Verification items for the finished model (mm, model axes). Face numbers are marked on the shaded views. A direction names the side the tool comes from. Round coordinates to 2 decimals unless told otherwise and drop trailing zeros. Write each loop counter-clockwise with the first axis right and the second up, starting at its lowest first coordinate (ties: lowest second). Pieces come first, ordered by that corner, then holes. Notation, with made-up numbers: M 18,-9 L 63,-9 A28 cw 63,18 Z; hole C 7,2 d3. An arc over 180 degrees is marked long. One line per question, with ' | ' between items. Start each with the question number.
Q1. Gauge pin test, flat ends, axial feed: pin 1 (4 mm diameter, centred on x = 1.5, y = -3, fed in from +Z); pin 2 (10 mm diameter, centred on x = 27, y = 22.5, fed in from -Z); pin 3 (6 mm diameter, centred on y = 29, z = -5.5, fed in from +X). Record the tip position at first contact, or that the pin passes through.
Q2. Cross-section at B-B (z = 14.5). Record the boundary of the cut face in (x, y).
Q3. Release check for a two-part mould opening along X. For the marked faces 1 and 2 record: released by +X, released by -X, zero draft, split by the parting line, or undercut.
Q4. Cross-section at D-D (z = 0). Record the boundary of the cut face in (x, y).
Q5. Cross-section at A-A (y = 0). Record the boundary of the cut face in (x, z).
Q6. Cross-section at C-C (x = -26). Record the boundary of the cut face in (y, z), then the cut area to 3 significant figures.
Q7. Thickness scan on line 1 along Z through (x, y) = (-26, 32.75); line 2 along X through (y, z) = (34, 0); line 3 along Z through (x, y) = (-13, 0). Record the ranges inside material, lowest first. Write a range as from..to.
Q8. Tool access check on the marked faces 3 and 4. Record the directions out of +Z, -Z, +X, -X, +Y, -Y that give a thin tool (end or side, any length) a straight path to the whole face; none if there is none.
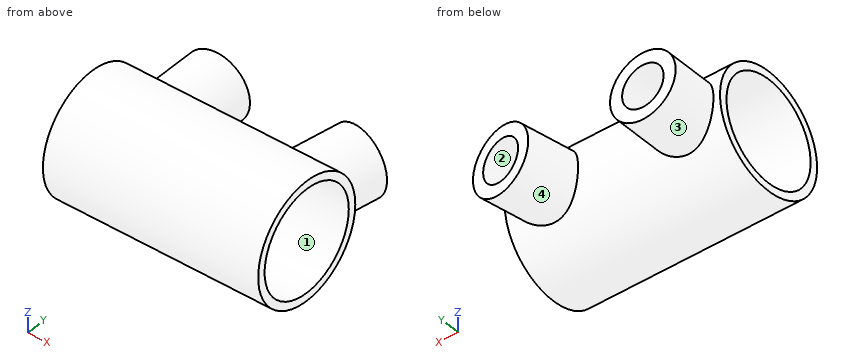
Autodesk Inventor part; units mm, degrees
ref_plane "Work Plane1" through (0, 40, 0) normal (0, 1, 0) x (-1, 0, 0)
ref_plane "Work Plane3" through (25, 40, 22.5) normal (0.1736, 0.9848, 0) x (0, 0, -1)
ref_plane "YZ Plane" through (0, 0, 0) normal (1, 0, 0) x (0, 1, 0)
sketch "Sketch1" plane through (0, 0, 0) normal (1, 0, 0) x (0, 1, 0)
  circle A0 centre (0, 0) radius 19.5
  circle A1 centre (0, 0) radius 22.5
  dimension "d0" = 39
  dimension "d1" = 45
extrude "Extrusion1" add sketch "Sketch1" along normal mid plane 82
ref_plane "Work Plane1" through (0, 40, 0) normal (0, 1, 0) x (-1, 0, 0)
sketch "Sketch2" plane through (0, 40, 0) normal (0, 1, 0) x (-1, 0, 0)
  circle A0 centre (26, 0) radius 12.5
  circle A1 centre (26, 0) radius 7.9
  line L0 (41, -22.5) -> (41, 22.5)
  point P0 (0, 0)
  dimension "d6" = 25
  dimension "d7" = 15.8
  dimension "d19" = 15
extrude "Extrusion2" add sketch "Sketch2" against normal up to surface
sketch "Sketch3" plane through (0, 40, 0) normal (0, 1, 0) x (-1, 0, 0)
  line L0 (41, 22.5) -> (-41, 22.5)
  line L1 (-25, 22.5) -> (-25, -21.8926)
  line L2 (41, 22.5) -> (-41, 22.5)
  point P0 (0, 0)
  dimension "d16" = 25
ref_plane "Work Plane3" through (25, 40, 22.5) normal (0.1736, 0.9848, 0) x (0, 0, -1)
sketch "Sketch4" plane through (25, 40, 22.5) normal (0.1736, 0.9848, 0) x (0, 0, -1)
  ellipse E0 centre (22.5, 50.2252) end of major axis (14.6, 50.2252) minor radius 7.78
  circle A0 centre (22.5, -3.7748) radius 7.9
  circle A1 centre (22.5, -3.7748) radius 12.5
  ellipse E1 centre (22.5, 50.2252) end of major axis (10, 50.2252) minor radius 12.3101
  point P0 (22.5, 17.6743)
  dimension "d11" = 54
  dimension "d12" = 15.8
  dimension "d13" = 25
extrude "Extrusion3" add sketch "Sketch4" against normal up to surface contours A1
properties part number "JuntaRodilla" material "PLA"
Determined:
1) pin 1: stops at z = 22.48 | pin 2: stops at z = -14.14 | pin 3: stops at x = 39.51
2) outline: M -41,-17.2 L 41,-17.2 L 41,-13.04 L -41,-13.04 Z; M -41,13.04 L 41,13.04 L 41,17.2 L -41,17.2 Z
3) face 1: zero draft | face 2: undercut
4) outline: M -41,-22.5 L 41,-22.5 L 41,-19.5 L -41,-19.5 Z; M -41,19.5 L 41,19.5 L 41,22.5 L 38.44,22.5 L 41.03,37.17 L 36.5,37.97 L 33.77,22.5 L 17.73,22.5 L 20.94,40.72 L 16.41,41.52 L 13.05,22.5 L -13.5,22.5 L -13.5,40 L -18.1,40 L -18.1,22.5 L -33.9,22.5 L -33.9,40 L -38.5,40 L -38.5,22.5 L -41,22.5 Z
5) outline: M -41,-22.5 L 41,-22.5 L 41,-19.5 L -41,-19.5 Z; M -41,19.5 L 41,19.5 L 41,22.5 L -41,22.5 Z
6) outline: M 18.71,-12.5 L 40,-12.5 L 40,-7.9 L 21.07,-7.9 A22.5 ccw 21.07,7.9 L 40,7.9 L 40,12.5 L 18.71,12.5 A22.5 ccw long Z; hole C 0,0 d39 | area: 580 mm²
7) line 1: z = -12.5..-7.9, 7.9..12.5 | line 2: x = -38.5..-33.9, -18.1..-13.5, 15.08..19.75, 35.8..40.47 | line 3: z = -22.5..-19.5, 19.5..22.5
8) face 3: +Y | face 4: none
